```python
from build123d import *

# Parameters (mm, degrees)
F0_W     = 3
F0_H     = 610
F1_DEPTH = 600
F2_W     = 606
F2_H     = 616
F3_DEPTH = 3


with BuildPart() as f1:
    # F0 (on Top) → F1 (new body)
    with BuildSketch(Plane.XY):
        Polygon((304.217247, 285.197261), (-301.782753, 285.197261), (-301.782753, 282.197261), (-298.782753, 282.197261), (301.217247, 282.197261), (304.217247, 282.197261), align=None)
        with Locations((-300.282753, -22.802739)):
            Rectangle(F0_W, F0_H)
        with Locations((302.717247, -22.802739)):
            Rectangle(F0_W, F0_H)
        Polygon((-298.782753, -327.802739), (-301.782753, -327.802739), (-301.782753, -330.802739), (304.217247, -330.802739), (304.217247, -327.802739), (301.217247, -327.802739), align=None)
    extrude(amount=F1_DEPTH)

    # F2 (on face) → F3 (join)
    with BuildSketch(Plane.XY.offset(600)):
        with Locations((1.217247, -22.802739)):
            Rectangle(F2_W, F2_H)
    extrude(amount=F3_DEPTH)


solid = f1.part
```
For this review, take the finished solid that the model builds, in its own axes (mm). A direction names the side the tool comes from. Coordinates: 2 decimals unless noted, no trailing zeros. Write each loop counter-clockwise with the first axis right and the second up, starting at its lowest first coordinate (ties: lowest second). Pieces come first, ordered by that corner, then holes. Notation, with made-up numbers: (-5.75, -15.75) - (41.25, -15.75) arc R34 ccw to (41.25, 19.25) - close; hole circle Ø5 at (83, 17). An arc over 180 degrees is marked (long way). Put each result on its own line as item: value.
1. Wall thickness on probe 1 along X at (y, z) = (21, 270); probe 2 along Y at (x, z) = (-76, 190); probe 3 along Z at (x, y) = (-52, -222): over which ranges is each line inside the solid? List them lowest first.
Values found:
probe 1: -301.78 to -298.78, 301.22 to 304.22
probe 2: -330.8 to -327.8, 282.2 to 285.2
probe 3: 600 to 603
2. Add section B-B, the plane z = 122. Give the boundary of the cut face in (x, y), then the cut area to 3 significant figures.
Values found:
outline: (-301.78, -330.8) - (304.22, -330.8) - (304.22, 285.2) - (-301.78, 285.2) - close; hole (-298.78, -327.8) - (301.22, -327.8) - (301.22, 282.2) - (-298.78, 282.2) - close
area: 7,300 mm²
3. Add section A-A, the plane y = 14. Give the boundary of the cut face in (x, z), then the cut area to 3 significant figures.
Values found:
outline: (-301.78, 0) - (-298.78, 0) - (-298.78, 600) - (301.22, 600) - (301.22, 0) - (304.22, 0) - (304.22, 603) - (-301.78, 603) - close
area: 5,420 mm²
4. For pin 1 (5 mm diameter, centred on x = 199, y = -150.5, fed in from -Z), flat-tipped, find the tip position at first contact; note if it passes through.
Values found:
pin 1: z = 600
5. Machinability: for faces 1 (the flat face through (301.217, -27, 296)), 2 (the flat face through (-3, -330.803, 297)), which of the approach directions +Z, -Z, +X, -X, +Y, -Y give a long, thin tool a straight path to every point of the face, cutting with its end or side? Answer none if there is none.
Values found:
face 1: -Z
face 2: +Z, -Z, +X, -X, -Y
6. Add section C-C, the plane x = 43. Give the boundary of the cut face in (y, z), then the cut area to 3 significant figures.
Values found:
outline: (-330.8, 0) - (-327.8, 0) - (-327.8, 600) - (282.2, 600) - (282.2, 0) - (285.2, 0) - (285.2, 603) - (-330.8, 603) - close
area: 5,450 mm²
7. Mouldability with a two-part tool opening along X and no side actions: class faces 3 (the flat face through (-3, 282.197, 296)), 4 (the flat face through (304.217, -27, 297)), 5 (the flat face through (-301.783, -27, 297)), 6 (the flat face through (5, -327.803, 296)) as released by +X, released by -X, zero draft, split by the parting line, or undercut.
Values found:
face 3: undercut
face 4: released by +X
face 5: released by -X
face 6: undercut
